from build123d import *

# Parameters (mm, degrees)
SKETCH1_W           = 35
SKETCH1_H           = 48
BOSS_EXTRUDE1_DEPTH = 2
SKETCH2_W           = 35
SKETCH2_H           = 48
SKETCH2_W_2         = 31
SKETCH2_H_2         = 44
BOSS_EXTRUDE2_DEPTH = 7.3
SKETCH3_W           = 10
SKETCH3_H           = 7
SKETCH3_W_2         = 5.25
SKETCH3_H_2         = 6.4
BOSS_EXTRUDE3_DEPTH = 6.1
CUT_EXTRUDE5_DEPTH  = 1
SKETCH10_W          = 31
SKETCH10_H          = 28.6
CUT_EXTRUDE6_DEPTH  = 31.586598372
BOSS_EXTRUDE4_START = 8.1
SKETCH8_R           = 1.45
BOSS_EXTRUDE4_DEPTH = 6
SKETCH12_W          = 6
SKETCH12_H          = 4
BOSS_EXTRUDE5_DEPTH = 3.5
SKETCH13_W          = 2
SKETCH13_H          = 2.8
CUT_EXTRUDE7_DEPTH  = 4


with BuildPart() as part:
    # Sketch1 → Boss-Extrude1 (new body)
    with BuildSketch(Plane(origin=(0, 0, 0), x_dir=(1, 0, 0), z_dir=(0, 1, 0))):
        Rectangle(SKETCH1_W, SKETCH1_H)
    extrude(amount=BOSS_EXTRUDE1_DEPTH)

    # Sketch2 → Boss-Extrude2 (add)
    with BuildSketch(Plane(origin=(0, 2, 0), x_dir=(1, 0, 0), z_dir=(0, 1, 0))):
        Rectangle(SKETCH2_W, SKETCH2_H)
        with Locations((0, 1)):
            Rectangle(SKETCH2_W_2, SKETCH2_H_2, mode=Mode.SUBTRACT)
    extrude(amount=BOSS_EXTRUDE2_DEPTH)

    # Sketch3 → Boss-Extrude3 (add)
    with BuildSketch(Plane(origin=(0, 2, 0), x_dir=(1, 0, 0), z_dir=(0, 1, 0))):
        with Locations((0, 19.5)):
            Rectangle(SKETCH3_W, SKETCH3_H)
        with Locations((-12.875, -17.8)):
            Rectangle(SKETCH3_W_2, SKETCH3_H_2)
        with Locations((12.875, -17.8)):
            Rectangle(SKETCH3_W_2, SKETCH3_H_2)
    extrude(amount=BOSS_EXTRUDE3_DEPTH)

    # Sketch6 → Cut-Extrude5 (cut)
    with BuildSketch(Plane(origin=(0, 0, -24), x_dir=(-1, 0, 0), z_dir=(0, 0, -1))):
        with BuildLine():
            ThreePointArc((-13.059411708, 9.3), (-10, 6.7), (-6.940588292, 9.3))
            Line((-6.940588292, 9.3), (-13.059411708, 9.3))
        make_face()
        with BuildLine():
            Line((13.059411708, 9.3), (6.940588292, 9.3))
            ThreePointArc((6.940588292, 9.3), (10, 6.7), (13.059411708, 9.3))
        make_face()
    extrude(amount=-CUT_EXTRUDE5_DEPTH, mode=Mode.SUBTRACT)

    # Sketch10 → Cut-Extrude6 (cut, through all)
    with BuildSketch(Plane(origin=(0, 2, 0), x_dir=(1, 0, 0), z_dir=(0, 1, 0))):
        with Locations((0, -0.3)):
            Rectangle(SKETCH10_W, SKETCH10_H)
    extrude(amount=-CUT_EXTRUDE6_DEPTH, mode=Mode.SUBTRACT)

    # Sketch8 → Boss-Extrude4 (add)
    with BuildSketch(Plane(origin=(0, 0, 0), x_dir=(1, 0, 0), z_dir=(0, 1, 0)).offset(BOSS_EXTRUDE4_START)):
        with Locations(Location((-12.55, -18.7, 0), (0, 0, 90))):
            Circle(SKETCH8_R)
        with Locations(Location((12.55, -18.7, 0), (0, 0, 270))):
            Circle(SKETCH8_R)
        with Locations(Location((0, 18.6, 0), (0, 0, 270))):
            Circle(SKETCH8_R)
    extrude(amount=BOSS_EXTRUDE4_DEPTH)

    # Sketch12 → Boss-Extrude5 (add)
    with BuildSketch(Plane.ZY.offset(17.5)):
        with Locations((0, 2)):
            Rectangle(SKETCH12_W, SKETCH12_H)
    boss_extrude5 = extrude(amount=BOSS_EXTRUDE5_DEPTH)

    # Sketch13 → Cut-Extrude7 (cut)
    with BuildSketch(Plane(origin=(0, 4, 0), x_dir=(1, 0, 0), z_dir=(0, 1, 0))):
        with Locations((-18.8, 0)):
            Rectangle(SKETCH13_W, SKETCH13_H)
    cut_extrude7 = extrude(amount=-CUT_EXTRUDE7_DEPTH, mode=Mode.SUBTRACT)

    # Mirror1: Boss-Extrude5, Cut-Extrude7 across plane
    add(boss_extrude5.mirror(Plane(origin=(0, 0, 0), x_dir=(0, 0, 1), z_dir=(1, 0, 0))))
    add(cut_extrude7.mirror(Plane(origin=(0, 0, 0), x_dir=(0, 0, 1), z_dir=(1, 0, 0))), mode=Mode.SUBTRACT)


solid = part.part
The listing builds one solid part. Answer for the finished solid, in the listing's coordinates (mm). A direction names the side the tool comes from. Coordinates: 2 decimals unless noted, no trailing zeros. Write each loop counter-clockwise with the first axis right and the second up, starting at its lowest first coordinate (ties: lowest second). Pieces come first, ordered by that corner, then holes. Notation, with made-up numbers: (0.25, 31.25) - (49.25, 31.25) arc R18 ccw to (49.25, 35.25) - close; hole circle Ø1 at (75.25, 86.5). An arc over 180 degrees is marked (long way). Return JSON: item names as keys, results as strings.
1. The part is cut by section A-A on y = 3. Count the separate pieces of the cut face and the enclosed holes in it, then the cut area to 3 significant figures.
Final values:
{"separate pieces": "1", "enclosed holes": "3", "area": "484 mm^2"}
2. The part is cut by section B-B on x = 0. Determine the outline of the cut face in (y, z).
Final values:
{"outline": "(0, -24) - (9.3, -24) - (9.3, -23) - (8.1, -23) - (8.1, -20.05) - (14.1, -20.05) - (14.1, -17.15) - (8.1, -17.15) - (8.1, -16) - (2, -16) - (2, -14) - (0, -14) - close; (0, 14.6) - (2, 14.6) - (2, 21) - (9.3, 21) - (9.3, 24) - (0, 24) - close"}
3. For a pull along Z with two mould halves and no side action, classify faces 1 (the face through (19, 2, 3)), 2 (the face through (-10.25, 5, 18)), 3 (the face through (21, 2, 0)) as +Z half, -Z half, draft (parallel to the pull), parting line (faces both ways), or undercut.
Final values:
{"face 1": "+Z half", "face 2": "undercut", "face 3": "draft"}
4. Each of these flat-tipped pins is pushed along its axis until it touches: pin 1 Ø3 at (y, z) = (2.5, -4) entering from -X; pin 2 Ø4.5 at (y, z) = (7, -3) entering from +X; pin 3 Ø3 at (y, z) = (5.5, -7.5) entering from -X; pin 4 Ø3 at (x, y) = (-7, 12) entering from -Z. Where does it stop, or does it pass through?
Final values:
{"pin 1": "x = -21", "pin 2": "x = 17.5", "pin 3": "x = -17.5", "pin 4": "through"}
5. Consider line 1 along X through (y, z) = (2.75, 4.5); line 2 along Z through (x, y) = (7.5, 2.25); line 3 along X through (y, z) = (4, -18). Determine where each line is inside the solid, lowest interval first.
Final values:
{"line 1": "-17.5 to -15.5, 15.5 to 17.5", "line 2": "-24 to -23, 21 to 24", "line 3": "-17.5 to -15.5, -5 to 5, 15.5 to 17.5"}
6. The part is cut by section D-D on z = 18.7. Determine the outline of the cut face in (x, y).
Final values:
{"outline": "(-17.5, 0) - (17.5, 0) - (17.5, 9.3) - (15.5, 9.3) - (15.5, 8.1) - (14, 8.1) - (14, 14.1) - (11.1, 14.1) - (11.1, 8.1) - (10.25, 8.1) - (10.25, 2) - (-10.25, 2) - (-10.25, 8.1) - (-11.1, 8.1) - (-11.1, 14.1) - (-14, 14.1) - (-14, 8.1) - (-15.5, 8.1) - (-15.5, 9.3) - (-17.5, 9.3) - close"}
7. The part is cut by section C-C on z = -10. Determine the outline of the cut face in (x, y).
Final values:
{"outline": "(-17.5, 0) - (-15.5, 0) - (-15.5, 9.3) - (-17.5, 9.3) - close; (15.5, 0) - (17.5, 0) - (17.5, 9.3) - (15.5, 9.3) - close"}
8. Which of the six approach directions +Z, -Z, +X, -X, +Y, -Y give full straight-line access (tool end or side, diameter ignored) to faces 4 (the face through (-0.1, 8.1, -20.3)), 5 (the face through (20, 4, 0)), 6 (the face through (-0.1, 9.3, -23.5)), 7 (the face through (-20, 4, 0)), 8 (the face through (0, 1, -14))?
Final values:
{"face 4": "+Y", "face 5": "+Z, -Z, +X, +Y", "face 6": "-Z, +X, -X, +Y", "face 7": "+Z, -Z, -X, +Y", "face 8": "+Y, -Y"}
